Input: part model. Units: mm. Frame: model coordinates. A direction names the side the tool comes from. Give positions to 0.01 mm unless a question says otherwise; leave off trailing zeros. Order: outer loops, then holes, each group sorted by start corner. A loop starts at its lowest first (then second) coordinate and runs counter-clockwise, first axis right, second up. Notation, with made-up numbers: (71, -36.75) - (88, -36.75) arc R21 cw to (88, -1.75) - close; hole circle Ø9 at (-19.75, -39). An arc over 180 degrees is marked (long way). Answer in a Markdown table with one row per item. Add a question column.
1. Section query D-D on z = 17. Return loops of the section in (x, y).
2. Section query A-A on x = -19. Return loops of the section in (y, z).
3. Contact query for flat-ended pins moving along their axis: pin 1 (4 mm diameter, centred on x = -16.5, z = 31.5, fed in from +Y); pin 2 (3 mm diameter, centred on y = 37.5, z = 7.5, fed in from -X); pin 3 (2 mm diameter, centred on x = -16.5, y = 51.5, fed in from +Z). Output: stop coordinate, or through.
4. Section query C-C on x = -4.5. Return loops of the section in (y, z), and give its area (3 significant figures).
5. Access query for faces 4 (the face through (-20.8, 57.3, 3.2)), 5 (the face through (-16, 42, 6.35)). Directions: +Z, -Z, +X, -X, +Y, -Y. A direction counts if a zero-diameter tool reaches every point of the face in a straight line with its end or side. Return the directions, or none.
6. Section query B-B on y = 57.15. Return loops of the section in (x, z).
7. Ray query, line 1 (Z direction, x = -14.5, y = 69.5). Return the intervals inside material, ascending. Write a range as [from, to].
8. Mould query, pull axis Y, two halves, no side actions, for faces 1 (the face through (-16.87, 4.901, 36.572)), 2 (the face through (-17.18, 29.53, 3.22)), 3 (the face through (-33.274, 27, 5)). Classes: released by +Y, released by -Y, zero draft, split by the parting line, or undercut.
```python
from build123d import *

# Parameters (mm, degrees)
F1_DEPTH = 33.274
F2_R     = 6.35
F3_R     = 5.08
F4_R     = 4.1656
F5_DEPTH = 6.351
F6_R     = 4.1656
F7_DEPTH = 6.351


with BuildPart() as f1:
    # F0 (on Right) → F1 (new body)
    with BuildSketch(Plane.YZ):
        Polygon((0, 38.1), (0, 0), (76.2, 0), (76.2, 6.35), (6.35, 6.35), (6.35, 38.1), align=None)
    extrude(amount=-F1_DEPTH)

    # F2
    f2_edges = [f1.edges().sort_by_distance(p)[0] for p in [
        (-16.637, 6.35, 6.35),
    ]]
    fillet(f2_edges, radius=F2_R)

    # F3
    f3_edges = [f1.edges().sort_by_distance(p)[0] for p in [
        (-16.637, 6.35, 38.1),
        (-16.637, 76.2, 6.35),
    ]]
    fillet(f3_edges, radius=F3_R)

    # F4 (on face) → F5 (cut, through all)
    with BuildSketch(Plane(origin=(0, 6.35, 0), x_dir=(-1, 0, 0), z_dir=(0, 1, 0))):
        with Locations((16.637, 22.225)):
            Circle(F4_R)
    extrude(amount=-F5_DEPTH, mode=Mode.SUBTRACT)

    # F6 (on face) → F7 (cut, through all)
    with BuildSketch(Plane.XY.offset(6.35)):
        with Locations((-16.637, 25.4)):
            Circle(F6_R)
        with Locations((-16.637, 57.15)):
            Circle(F6_R)
    extrude(amount=-F7_DEPTH, mode=Mode.SUBTRACT)


solid = f1.part
```
Answer:
| question | item | result |
|---|---|---|
| 1 | outline | (-33.27, 0) - (0, 0) - (0, 6.35) - (-33.27, 6.35) - close |
| 2 | outline | (0, 0) - (21.97, 0) - (21.97, 6.35) - (12.7, 6.35) arc R6.35 cw to (6.35, 12.7) - (6.35, 18.79) - (0, 18.79) - close; (0, 25.66) - (6.35, 25.66) - (6.35, 33.02) arc R5.08 ccw to (1.27, 38.1) - (0, 38.1) - close; (28.83, 0) - (53.72, 0) - (53.72, 6.35) - (28.83, 6.35) - close; (60.58, 0) - (76.2, 0) - (76.2, 1.27) arc R5.08 ccw to (71.12, 6.35) - (60.58, 6.35) - close |
| 3 | pin 1 | stops at y = 6.35 |
| 3 | pin 2 | stops at x = -33.27 |
| 3 | pin 3 | stops at z = 6.35 |
| 4 | outline | (0, 0) - (76.2, 0) - (76.2, 1.27) arc R5.08 ccw to (71.12, 6.35) - (12.7, 6.35) arc R6.35 cw to (6.35, 12.7) - (6.35, 33.02) arc R5.08 ccw to (1.27, 38.1) - (0, 38.1) - close |
| 4 | area | 683 mm² |
| 5 | face 4 | +Z, -Z |
| 5 | face 5 | +Z, +X, -X, +Y |
| 6 | outline | (-33.27, 0) - (-20.8, 0) - (-20.8, 6.35) - (-33.27, 6.35) - close; (-12.47, 0) - (0, 0) - (0, 6.35) - (-12.47, 6.35) - close |
| 7 | line 1 | z = [0, 6.35] |
| 8 | face 1 | released by +Y |
| 8 | face 2 | undercut |
| 8 | face 3 | zero draft |
